from build123d import *

# Parameters (mm, degrees)
F0_R     = 3
F0_W     = 0.793037466
F0_H     = 2.9075266591
F0_H_2   = 4.0467378773
F0_R_2   = 2
F1_DEPTH = 3


with BuildPart() as f1:
    # F0 (on Top) → F1 (new body)
    with BuildSketch(Plane.XY):
        with BuildLine():
            Line((-60, 5), (-60, -5))
            Line((-60, -5), (-4.8989794856, -5))
            ThreePointArc((-4.8989794856, -5), (-7, 0), (-4.8989794856, 5))
            Line((-4.8989794856, 5), (-52, 5))
            Line((-52, 5), (-52, 3))
            Line((-52, 3), (-56, 3))
            Line((-56, 3), (-56, 5))
            Line((-56, 5), (-60, 5))
        make_face()
        with Locations((-30, 0)):
            Circle(F0_R, mode=Mode.SUBTRACT)
        with BuildLine():
            ThreePointArc((7, 0), (6.4534043883, -2.7117470016), (4.8989794856, -5))
            Line((4.8989794856, -5), (60, -5))
            Line((60, -5), (60, 5))
            Line((60, 5), (59, 5))
            ThreePointArc((59, 5), (53, -1), (47, 5))
            Line((47, 5), (4.8989794856, 5))
            ThreePointArc((4.8989794856, 5), (6.4534043883, 2.7117470016), (7, 0))
        make_face()
        Polygon((22.4301818638, -3.8345400244), (21.5614188895, -3.8345400244), (21.2859777549, -2.9291625186), (19.8996184492, -2.9291625186), (19.6241773147, -3.8345400244), (18.7554143404, -3.8345400244), (20.0976697786, -0.0166429689), (21.0829335349, -0.0166429689), align=None, mode=Mode.SUBTRACT)
        with Locations((24.8679607269, -2.3807766948)):
            Rectangle(F0_W, F0_H, mode=Mode.SUBTRACT)
        with BuildLine():
            add(Edge.make_bspline(
                [(27.7725748665, -3.8399489893), (27.576187834, -3.8869653763), (27.277446543, -3.8869653763)],
                knots=[0, 0, 0, 1, 1, 1], degree=2))
            add(Edge.make_bspline(
                [(27.277446543, -3.8869653763), (25.9202124328, -3.8869653763), (25.9202124328, -2.3965875152)],
                knots=[0, 0, 0, 1, 1, 1], degree=2))
            add(Edge.make_bspline(
                [(25.9202124328, -2.3965875152), (25.9202124328, -1.6551432527), (26.2892702672, -1.2640334846)],
                knots=[0, 0, 0, 1, 1, 1], degree=2))
            add(Edge.make_bspline(
                [(26.2892702672, -1.2640334846), (26.6583281016, -0.8729237165), (27.3473470122, -0.8729237165)],
                knots=[0, 0, 0, 1, 1, 1], degree=2))
            add(Edge.make_bspline(
                [(27.3473470122, -0.8729237165), (27.8516289686, -0.8729237165), (28.252724518, -1.0701428974)],
                knots=[0, 0, 0, 1, 1, 1], degree=2))
            Line((28.252724518, -1.0701428974), (28.0180586571, -1.6842684482))
            add(Edge.make_bspline(
                [(28.0180586571, -1.6842684482), (27.8308252575, -1.6085429399), (27.6698045338, -1.5602783302)],
                knots=[0, 0, 0, 1, 1, 1], degree=2))
            add(Edge.make_bspline(
                [(27.6698045338, -1.5602783302), (27.5087838101, -1.5120137206), (27.3473470122, -1.5120137206)],
                knots=[0, 0, 0, 1, 1, 1], degree=2))
            add(Edge.make_bspline(
                [(27.3473470122, -1.5120137206), (26.7282285708, -1.5120137206), (26.7282285708, -2.3915946246)],
                knots=[0, 0, 0, 1, 1, 1], degree=2))
            add(Edge.make_bspline(
                [(26.7282285708, -2.3915946246), (26.7282285708, -3.2445467785), (27.3473470122, -3.2445467785)],
                knots=[0, 0, 0, 1, 1, 1], degree=2))
            add(Edge.make_bspline(
                [(27.3473470122, -3.2445467785), (27.576187834, -3.2445467785), (27.7713266438, -3.1833838679)],
                knots=[0, 0, 0, 1, 1, 1], degree=2))
            add(Edge.make_bspline(
                [(27.7713266438, -3.1833838679), (27.9664654537, -3.1222209574), (28.1611881893, -2.9915736518)],
                knots=[0, 0, 0, 1, 1, 1], degree=2))
            Line((28.1611881893, -2.9915736518), (28.1611881893, -3.6706067812))
            add(Edge.make_bspline(
                [(28.1611881893, -3.6706067812), (27.968961899, -3.7929326023), (27.7725748665, -3.8399489893)],
                knots=[0, 0, 0, 1, 1, 1], degree=2))
        make_face(mode=Mode.SUBTRACT)
        with BuildLine():
            add(Edge.make_bspline(
                [(30.7283661353, -3.8362043213), (30.4920359776, -3.8869653763), (30.150855116, -3.8869653763)],
                knots=[0, 0, 0, 1, 1, 1], degree=2))
            add(Edge.make_bspline(
                [(30.150855116, -3.8869653763), (29.4493539787, -3.8869653763), (29.0540834684, -3.499184202)],
                knots=[0, 0, 0, 1, 1, 1], degree=2))
            add(Edge.make_bspline(
                [(29.0540834684, -3.499184202), (28.6588129581, -3.1114030276), (28.6588129581, -2.4015804059)],
                knots=[0, 0, 0, 1, 1, 1], degree=2))
            add(Edge.make_bspline(
                [(28.6588129581, -2.4015804059), (28.6588129581, -1.6709540731), (29.0241261245, -1.2719388948)],
                knots=[0, 0, 0, 1, 1, 1], degree=2))
            add(Edge.make_bspline(
                [(29.0241261245, -1.2719388948), (29.3894392909, -0.8729237165), (30.034354334, -0.8729237165)],
                knots=[0, 0, 0, 1, 1, 1], degree=2))
            add(Edge.make_bspline(
                [(30.034354334, -0.8729237165), (30.6501441817, -0.8729237165), (30.9934054143, -1.2236742851)],
                knots=[0, 0, 0, 1, 1, 1], degree=2))
            add(Edge.make_bspline(
                [(30.9934054143, -1.2236742851), (31.336666647, -1.5744248538), (31.336666647, -2.1935432952)],
                knots=[0, 0, 0, 1, 1, 1], degree=2))
            Line((31.336666647, -2.1935432952), (31.336666647, -2.5788280242))
            Line((31.336666647, -2.5788280242), (29.4618362054, -2.5788280242))
            add(Edge.make_bspline(
                [(29.4618362054, -2.5788280242), (29.4751505805, -2.916680292), (29.6623839801, -3.106410137)],
                knots=[0, 0, 0, 1, 1, 1], degree=2))
            add(Edge.make_bspline(
                [(29.6623839801, -3.106410137), (29.8496173797, -3.2961399819), (30.1874696475, -3.2961399819)],
                knots=[0, 0, 0, 1, 1, 1], degree=2))
            add(Edge.make_bspline(
                [(30.1874696475, -3.2961399819), (30.4504285554, -3.2961399819), (30.6842622678, -3.2416342589)],
                knots=[0, 0, 0, 1, 1, 1], degree=2))
            add(Edge.make_bspline(
                [(30.6842622678, -3.2416342589), (30.9180959803, -3.1871285359), (31.1727334038, -3.0672991601)],
                knots=[0, 0, 0, 1, 1, 1], degree=2))
            Line((31.1727334038, -3.0672991601), (31.1727334038, -3.6814247109))
            add(Edge.make_bspline(
                [(31.1727334038, -3.6814247109), (30.9646962931, -3.7854432663), (30.7283661353, -3.8362043213)],
                knots=[0, 0, 0, 1, 1, 1], degree=2))
        make_face(mode=Mode.SUBTRACT)
        with Locations((23.2427748181, -1.8111710857)):
            Rectangle(F0_W, F0_H_2, mode=Mode.SUBTRACT)
        with BuildLine():
            add(Edge.make_bspline(
                [(24.8692089496, -0.5658609411), (24.4373239078, -0.5658609411), (24.4373239078, -0.1755833214)],
                knots=[0, 0, 0, 1, 1, 1], degree=2))
            add(Edge.make_bspline(
                [(24.4373239078, -0.1755833214), (24.4373239078, 0.2121978529), (24.8692089496, 0.2121978529)],
                knots=[0, 0, 0, 1, 1, 1], degree=2))
            add(Edge.make_bspline(
                [(24.8692089496, 0.2121978529), (25.3010939914, 0.2121978529), (25.3010939914, -0.1755833214)],
                knots=[0, 0, 0, 1, 1, 1], degree=2))
            add(Edge.make_bspline(
                [(25.3010939914, -0.1755833214), (25.3010939914, -0.3603202757), (25.1933307681, -0.4630906084)],
                knots=[0, 0, 0, 1, 1, 1], degree=2))
            add(Edge.make_bspline(
                [(25.1933307681, -0.4630906084), (25.0855675447, -0.5658609411), (24.8692089496, -0.5658609411)],
                knots=[0, 0, 0, 1, 1, 1], degree=2))
        make_face(mode=Mode.SUBTRACT)
        with BuildLine():
            Line((4.8989794856, -5), (-4.8989794856, -5))
            ThreePointArc((-4.8989794856, -5), (0, -7), (4.8989794856, -5))
        make_face()
        with BuildLine():
            ThreePointArc((-4.8989794856, 5), (-7, 0), (-4.8989794856, -5))
            Line((-4.8989794856, -5), (4.8989794856, -5))
            ThreePointArc((4.8989794856, -5), (6.4534043883, -2.7117470016), (7, 0))
            ThreePointArc((7, 0), (6.4534043883, 2.7117470016), (4.8989794856, 5))
            Line((4.8989794856, 5), (-4.8989794856, 5))
        make_face()
        Circle(F0_R_2, mode=Mode.SUBTRACT)
        with BuildLine():
            ThreePointArc((4.8989794856, 5), (0, 7), (-4.8989794856, 5))
            Line((-4.8989794856, 5), (4.8989794856, 5))
        make_face()
    extrude(amount=F1_DEPTH)


solid = f1.part
Work out the finished part from the listing and answer in its coordinate system (mm). A direction names the side the tool comes from. Round coordinates to 2 decimals unless told otherwise and drop trailing zeros. Write each loop counter-clockwise with the first axis right and the second up, starting at its lowest first coordinate (ties: lowest second). Pieces come first, ordered by that corner, then holes. Notation, with made-up numbers: (31.5, 52) -> (42.5, 52) arc R27 cw to (42.5, 87) -> close; hole circle Ø1 at (54.25, 48). An arc over 180 degrees is marked (long way). Write each question's results on one line, items separated by ' | '.
Item 1: A cutting plane is placed at B-B, the plane x = -30. Determine the outline of the cut face in (y, z), plus the area to 3 significant figures.
Result set:
outline: (-5, 0) -> (-3, 0) -> (-3, 3) -> (-5, 3) -> close; (3, 0) -> (5, 0) -> (5, 3) -> (3, 3) -> close | area: 12.0 mm^2
Item 2: Which of the six approach directions +Z, -Z, +X, -X, +Y, -Y give full straight-line access (tool end or side, diameter ignored) to faces 4 (the face through (-33, -5, 1)), 5 (the face through (25.264, -2, 1)), 6 (the face through (-56, 4, 1)), 7 (the face through (26, 5, 1)), 8 (the face through (-58, 5, 1))?
Result set:
face 4: +Z, -Z, -X, -Y | face 5: +Z, -Z | face 6: +Z, -Z, +Y | face 7: +Z, -Z, +X, +Y | face 8: +Z, -Z, -X, +Y
Item 3: The mould has two halves that part along X. Classify faces 1 (the face through (53, -1, 1)), 2 (the face through (32, -5, 1)), 3 (the face through (0, 7, 1)): +X half, -X half, draft (parallel to the pull), parting line (faces both ways), or undercut.
Result set:
face 1: undercut | face 2: draft | face 3: parting line
Item 4: A cutting plane is placed at A-A, the plane x = 0. Determine the outline of the cut face in (y, z).
Result set:
outline: (-7, 0) -> (-2, 0) -> (-2, 3) -> (-7, 3) -> close; (2, 0) -> (7, 0) -> (7, 3) -> (2, 3) -> close
Item 5: A cutting plane is placed at D-D, the plane x = 53. Determine the outline of the cut face in (y, z), plus the area to 3 significant figures.
Result set:
outline: (-5, 0) -> (-1, 0) -> (-1, 3) -> (-5, 3) -> close | area: 12.0 mm^2
Item 6: Flat-ended cylindrical pins translate along their axes: P1, Ø0.6, axis at x = 23.5, z = 1, coming from the -Y side; P2, Ø1.1, axis at x = 20.5, z = 2, coming from the +Y side; P3, Ø2, axis at x = -40, y = -5, coming from the -Z side. Find the tip coordinate at first contact, or state that the pin passes through.
Result set:
P1: y = -5 | P2: y = 5 | P3: z = 0
Item 7: Find the intervals of material crossed by line 1 along X through (y, z) = (1.5, 2.25); line 2 along Y through (x, z) = (-30, 1.25); line 3 along Y through (x, z) = (-15, 2.75), in increasing order. Write a range as [from, to].
Result set:
line 1: [-60, -32.6], [-27.4, -1.32], [1.32, 48.13], [57.87, 60] | line 2: [-5, -3], [3, 5] | line 3: [-5, 5]
Item 8: A cutting plane is placed at C-C, the plane z = 1.8. Count the separate pieces of the cut face and the enclosed holes in it, plus the area to 3 significant figures.
Result set:
separate pieces: 1 | enclosed holes: 8 | area: 1,100 mm^2
